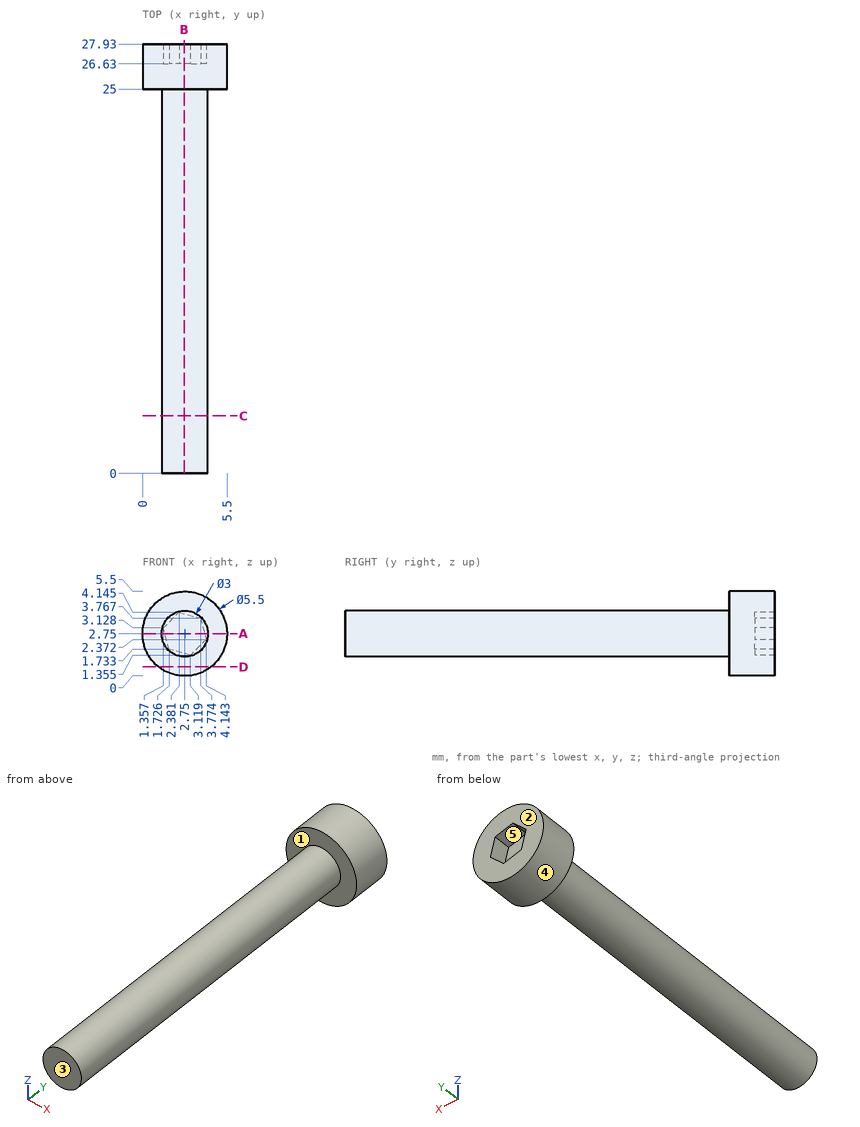
Input: dimensioned drawing with shaded views. Units: mm. Origin: part minimum x, y, z. A direction names the side the tool comes from. Round coordinates to 2 decimals unless told otherwise and drop trailing zeros. Loops run counter-clockwise (first coordinate to the right, second up) from the corner with the lowest first, then second, coordinate; pieces in that order, holes last. Notation, with made-up numbers: (-39, 29.5) -> (7, 29.5) arc R28 cw to (7, 61.5) -> close; hole circle Ø2 at (-18.75, -18.75). An arc over 180 degrees is marked (long way). Answer as a JSON object with one key per item and string values. Group by question number.
Q1. Section query B-B (x = 2.7). Output: boundary loops of the cut face in (y, z).
Q2. Section query C-C (y = 3.75). Output: boundary loops of the cut face in (x, z).
Q3. Contact query for flat-ended pins moving along their axis: P1, Ø0.8, axis at x = 3.5, z = 3, coming from the +Y side; P2, Ø3, axis at x = 1.5, z = 2.5, coming from the -Y side; P3, Ø1, axis at y = 19.5, z = 2.5, coming from the -X side. Output: stop coordinate, or through.
Q4. Access query for the marked faces 1 and 2. Directions: +Z, -Z, +X, -X, +Y, -Y. A direction counts if a zero-diameter tool reaches every point of the face in a straight line with its end or side. Return the directions, or none.
Q5. Ray query, line 1 (Y direction, x = 5.1, z = 1.45); line 2 (Y direction, x = 3.3, z = 2.7); line 3 (Z direction, x = 2.1, y = 16.25). Return the intervals inside material, ascending. Write a range as from..to.
Q6. Section query A-A (z = 2.75). Output: boundary loops of the cut face in (x, y).
Q7. Mould query, pull axis Z, two halves, no side actions, for the marked faces 3, 4 and 5. Classes: pulls with the +Z half, pulls with the -Z half, needs draft (parallel to the pull), parting line crosses it, or undercut.
Q8. Section query D-D (z = 0.6). Output: boundary loops of the cut face in (x, y) (1 decimal).
Completed:
{
 "1": {"outline": "(0, 1.25) -> (25, 1.25) -> (25, 0) -> (27.93, 0) -> (27.93, 1.47) -> (26.63, 1.47) -> (26.63, 4.06) -> (27.93, 4.06) -> (27.93, 5.5) -> (25, 5.5) -> (25, 4.25) -> (0, 4.25) -> close"},
 "2": {"outline": "circle Ø3 at (2.75, 2.75)"},
 "3": {"P1": "y = 26.63", "P2": "y = 0", "P3": "x = 1.25"},
 "4": {"face 1": "-Y", "face 2": "+Z, -Z, +X, -X, +Y"},
 "5": {"line 1": "25..27.93", "line 2": "0..26.63", "line 3": "1.4..4.1"},
 "6": {"outline": "(0, 25) -> (1.25, 25) -> (1.25, 0) -> (4.25, 0) -> (4.25, 25) -> (5.5, 25) -> (5.5, 27.93) -> (4.04, 27.93) -> (4.04, 26.63) -> (1.46, 26.63) -> (1.46, 27.93) -> (0, 27.93) -> close"},
 "7": {"face 3": "needs draft", "face 4": "parting line crosses it", "face 5": "undercut"},
 "8": {"outline": "(1, 25) -> (4.5, 25) -> (4.5, 27.9) -> (1, 27.9) -> close"}
}
